```python
from build123d import *

# Parameters (mm, degrees)
BOSS_EXTRUDE1_DEPTH   = 27.432
BOSS_EXTRUDE2_DEPTH   = 5.08
SKETCH4_R             = 1.524
CUT_EXTRUDE1_DEPTH    = 2.286
SKETCH4_4_R           = 1.524
CUT_EXTRUDE2_DEPTH    = 63.630575033
BOSS_EXTRUDE3_DEPTH   = 3.81
FILLET1_R             = 2.54
CHAMFER3_SIZE         = 1.27
CHAMFER4_SIZE         = 0.254
SKETCH8_W             = 101.6
SKETCH8_H             = 44.45
CUT_EXTRUDE3_DEPTH    = 5.08
CHAMFER5_SIZE         = 1.27
BOSS_EXTRUDE4_DEPTH   = 6.096
FILLET2_R             = 1.27
CUT_EXTRUDE4_DEPTH    = 15.24
MIRROR3_COPY_1_DEPTH  = 15.24
CHAMFER7_SIZE         = 0.381
SKETCH19_W            = 135.869666512
SKETCH19_H            = 67.345799606
CUT_EXTRUDE9_DEPTH    = 31.242
BOSS_EXTRUDE6_DEPTH   = 20.32
SKETCH21_W            = 80.01
SKETCH21_H            = 52.07
BOSS_EXTRUDE7_DEPTH   = 3.81
FILLET3_R             = 2.54
CHAMFER8_SIZE         = 1.27
BOSS_EXTRUDE8_DEPTH   = 10.16
BOSS_EXTRUDE10_DEPTH  = 5.08
MIRROR13_COPY_1_DEPTH = 10.16
MIRROR13_COPY_2_DEPTH = 5.08
SKETCH27_W            = 107.092264377
SKETCH27_H            = 185.22400122
CUT_EXTRUDE11_DEPTH   = 177.054251014
SKETCH28_W            = 133.557103753
SKETCH28_H            = 91.2241148
CUT_EXTRUDE12_DEPTH   = 45.72


with BuildPart() as part:
    # Sketch1 → Boss-Extrude1 (new body)
    with BuildSketch(Plane(origin=(10.858740921, 0, 0), x_dir=(1, 0, 0), z_dir=(0, 0, 1))):
        Polygon((-52.705, 25.4), (-52.705, 21.59), (48.895, 21.59), (48.895, -22.86), (-52.705, -22.86), (-52.705, -25.4), (52.705, -25.4), (52.705, 25.4), align=None)
    extrude(amount=BOSS_EXTRUDE1_DEPTH)

    # Sketch1<3> → Boss-Extrude2 (add)
    with BuildSketch(Plane(origin=(10.858740921, 0, 0), x_dir=(1, 0, 0), z_dir=(0, 0, 1))):
        Polygon((48.895, 21.59), (-52.705, 21.59), (-52.705, 13.97), (-6.985, 13.97), (-6.985, -6.35), (-52.705, -6.35), (-52.705, -22.86), (48.895, -22.86), align=None)
    extrude(amount=BOSS_EXTRUDE2_DEPTH)

    # Sketch4 → Cut-Extrude1 (cut)
    # profile 1 of 4: a face of its own
    with BuildSketch(Plane(origin=(10.858740921, 0, 5.08), x_dir=(1, 0, 0), z_dir=(0, 0, 1))):
        Polygon((-44.785877438, 21.59), (-47.924122562, 21.59), (-49.493245123, 18.8722), (-47.924122562, 16.1544), (-44.785877438, 16.1544), (-43.216754877, 18.8722), align=None)
        with Locations((-46.355, 18.8722)):
            Circle(SKETCH4_R, mode=Mode.SUBTRACT)
    # profile 2 of 4: a face of its own
    with BuildSketch(Plane(origin=(10.858740921, 0, 5.08), x_dir=(1, 0, 0), z_dir=(0, 0, 1))):
        Polygon((21.126640721, 16.1544), (17.988395597, 16.1544), (16.419273036, 18.8722), (17.988395597, 21.59), (21.126640721, 21.59), (22.695763282, 18.8722), align=None)
        with Locations((19.557518159, 18.8722)):
            Circle(SKETCH4_R, mode=Mode.SUBTRACT)
    # profile 3 of 4: a face of its own
    with BuildSketch(Plane(origin=(10.858740921, 0, 5.08), x_dir=(1, 0, 0), z_dir=(0, 0, 1))):
        Polygon((22.695763282, -18.8722), (21.126640721, -16.1544), (17.988395597, -16.1544), (16.419273036, -18.8722), (17.988395597, -21.59), (21.126640721, -21.59), align=None)
        with Locations((19.557518159, -18.8722)):
            Circle(SKETCH4_R, mode=Mode.SUBTRACT)
    # profile 4 of 4: a face of its own
    with BuildSketch(Plane(origin=(10.858740921, 0, 5.08), x_dir=(1, 0, 0), z_dir=(0, 0, 1))):
        Polygon((-49.493245123, -18.8722), (-47.924122562, -16.1544), (-44.785877438, -16.1544), (-43.216754877, -18.8722), (-44.785877438, -21.59), (-47.924122562, -21.59), align=None)
        with Locations((-46.355, -18.8722)):
            Circle(SKETCH4_R, mode=Mode.SUBTRACT)
    extrude(amount=-CUT_EXTRUDE1_DEPTH, mode=Mode.SUBTRACT)

    # Sketch4<4> → Cut-Extrude2 (cut, through all)
    with BuildSketch(Plane(origin=(10.858740921, 0, 5.08), x_dir=(1, 0, 0), z_dir=(0, 0, 1))):
        with Locations((-46.355, 18.8722)):
            Circle(SKETCH4_4_R)
        with Locations((19.557518159, 18.8722)):
            Circle(SKETCH4_4_R)
        with Locations((-46.355, -18.8722)):
            Circle(SKETCH4_4_R)
        with Locations((19.557518159, -18.8722)):
            Circle(SKETCH4_4_R)
    extrude(amount=-CUT_EXTRUDE2_DEPTH, mode=Mode.SUBTRACT)

    # Sketch7 → Boss-Extrude3 (add)
    with BuildSketch(Plane(origin=(10.858740921, 0, 27.432), x_dir=(1, 0, 0), z_dir=(0, 0, 1))):
        Polygon((-52.705, 25.4), (52.705, 25.4), (52.705, -25.4), (-52.705, -25.4), (-52.705, -6.35), (-46.355, -6.35), (-46.355, 6.35), (-52.705, 6.35), align=None)
    extrude(amount=BOSS_EXTRUDE3_DEPTH)

    # Fillet1
    fillet1_edges = [part.edges().sort_by_distance(p)[0] for p in [
        (63.563740921, 25.4, 15.621),
        (63.563740921, -25.4, 15.621),
        (10.858740921, -25.4, 31.242),
        (63.563740921, 0, 31.242),
        (10.858740921, 25.4, 31.242),
    ]]
    fillet(fillet1_edges, radius=FILLET1_R)

    # Chamfer3
    chamfer3_edges = [part.edges().sort_by_distance(p)[0] for p in [
        (-41.846259079, 13.97, 27.432),
        (-41.846259079, 6.35, 29.337),
        (-41.846259079, 21.59, 16.256),
        (-41.846259079, -14.605, 27.432),
        (-41.846259079, -6.35, 29.337),
        (-38.671259079, 6.35, 31.242),
        (-35.496259079, 0, 31.242),
        (-38.671259079, -6.35, 31.242),
        (-41.846259079, -22.86, 16.256),
    ]]
    chamfer(chamfer3_edges, length=CHAMFER3_SIZE)

    # Chamfer4
    chamfer4_edges = [part.edges().sort_by_distance(p)[0] for p in [
        (28.892259079, 18.8722, 0),
        (-37.020259079, -18.8722, 0),
        (28.892259079, -18.8722, 0),
        (-37.020259079, 18.8722, 0),
    ]]
    chamfer(chamfer4_edges, length=CHAMFER4_SIZE)

    # Sketch8 → Cut-Extrude3 (cut)
    with BuildSketch(Plane(origin=(10.858740921, 0, 5.08), x_dir=(1, 0, 0), z_dir=(0, 0, 1))):
        with Locations((-1.905, -0.635)):
            Rectangle(SKETCH8_W, SKETCH8_H)
    extrude(amount=-CUT_EXTRUDE3_DEPTH, mode=Mode.SUBTRACT)

    # Chamfer5
    chamfer5_edges = [part.edges().sort_by_distance(p)[0] for p in [
        (-41.846259079, -22.86, 2.54),
        (-41.846259079, 21.59, 2.54),
    ]]
    chamfer(chamfer5_edges, length=CHAMFER5_SIZE)

    # Sketch9 → Boss-Extrude4 (add)
    with BuildSketch(Plane(origin=(10.858740921, 0, 0), x_dir=(-1, 0, 0), z_dir=(0, 0, -1))):
        Polygon((-90.741259079, 28.1), (-80.741259079, 38.1), (102.458740921, 38.1), (112.458740921, 28.1), (112.458740921, -28.1), (102.458740921, -38.1), (-80.741259079, -38.1), (-90.741259079, -28.1), align=None)
    extrude(amount=BOSS_EXTRUDE4_DEPTH)

    # Fillet2
    fillet2_edges = [part.edges().sort_by_distance(p)[0] for p in [
        (9.588740921, -25.4, 0),
        (63.563740921, 0, 0),
        (9.588740921, 25.4, 0),
        (62.819792145, 24.656051224, 0),
        (62.819792145, -24.656051224, 0),
    ]]
    fillet(fillet2_edges, radius=FILLET2_R)

    # Sketch13 → Cut-Extrude4 (cut)
    with BuildSketch(Plane(origin=(-64.85, 64.85, 0), x_dir=(0, 0, 1), z_dir=(-0.7071067811865477, 0.7071067811865474, 0))):
        Polygon((-6.096, -44.901280605), (-6.096, -42.070807846), (0, -38.551280605), (0, -51.251280605), (-6.096, -47.731753364), align=None)
    cut_extrude4 = extrude(amount=-CUT_EXTRUDE4_DEPTH, mode=Mode.SUBTRACT)

    # Mirror2: Cut-Extrude4 across plane
    add(cut_extrude4.mirror(Plane.ZX), mode=Mode.SUBTRACT)

    # Mirror3: Cut-Extrude4 across plane
    add(cut_extrude4.mirror(Plane(origin=(0, 0, 0), x_dir=(0, 0, 1), z_dir=(1, 0, 0))), mode=Mode.SUBTRACT)

    # Mirror3 copy 1 sketch → Mirror3 copy 1 (cut)
    with BuildSketch(Plane(origin=(64.85, -64.85, 0), x_dir=(0, 0, 1), z_dir=(0.7071067811865477, -0.7071067811865474, 0))):
        Polygon((-6.096, -44.901280605), (-6.096, -42.070807846), (0, -38.551280605), (0, -51.251280605), (-6.096, -47.731753364), align=None)
    extrude(amount=-MIRROR3_COPY_1_DEPTH, mode=Mode.SUBTRACT)

    # Chamfer7
    chamfer7_edges = [part.edges().sort_by_distance(p)[0] for p in [
        (-99.845787271, 29.854212729, -3.048),
        (-93.354212729, 36.345787271, -3.048),
        (-99.845787271, -29.854212729, -3.048),
        (-93.354212729, -36.345787271, -3.048),
        (99.845787271, 29.854212729, -3.048),
        (93.354212729, 36.345787271, -3.048),
        (99.845787271, -29.854212729, -3.048),
        (93.354212729, -36.345787271, -3.048),
    ]]
    chamfer(chamfer7_edges, length=CHAMFER7_SIZE)

    # Sketch19 → Cut-Extrude9 (cut)
    with BuildSketch(Plane.XY.offset(31.242)):
        Rectangle(SKETCH19_W, SKETCH19_H)
    extrude(amount=-CUT_EXTRUDE9_DEPTH, mode=Mode.SUBTRACT)

    # Sketch20 → Boss-Extrude6 (add)
    with BuildSketch(Plane.XY):
        Polygon((65.405, 22.86), (65.405, -21.59), (-10.795, -21.59), (-10.795, -25.4), (69.215, -25.4), (69.215, 26.67), (-10.795, 26.67), (-10.795, 22.86), align=None)
    extrude(amount=BOSS_EXTRUDE6_DEPTH)

    # Sketch21 → Boss-Extrude7 (add)
    with BuildSketch(Plane.XY.offset(20.32)):
        with Locations((29.21, 0.635)):
            Rectangle(SKETCH21_W, SKETCH21_H)
    extrude(amount=BOSS_EXTRUDE7_DEPTH)

    # Fillet3
    fillet3_edges = [part.edges().sort_by_distance(p)[0] for p in [
        (29.21, -25.4, 0),
        (69.215, 0.635, 0),
        (69.215, -25.4, 12.065),
        (29.21, 26.67, 0),
        (69.215, 26.67, 12.065),
        (29.21, -25.4, 24.13),
        (69.215, 0.635, 24.13),
        (29.21, 26.67, 24.13),
    ]]
    fillet(fillet3_edges, radius=FILLET3_R)

    # Chamfer8
    chamfer8_edges = [part.edges().sort_by_distance(p)[0] for p in [
        (-10.795, 22.86, 10.16),
        (-10.795, -21.59, 10.16),
        (-10.795, 0.635, 20.32),
    ]]
    chamfer(chamfer8_edges, length=CHAMFER8_SIZE)

    # Sketch24 → Boss-Extrude8 (add)
    with BuildSketch(Plane.XY):
        Polygon((-90.762833521, 19.180603012), (-101.6, 8.343436534), (-101.6, 28.1), (-100.641115254, 29.058884746), align=None)
        Polygon((-92.558884746, 37.141115254), (-91.6, 38.1), (-71.843436534, 38.1), (-82.680603012, 27.262833521), align=None)
    boss_extrude8 = extrude(amount=BOSS_EXTRUDE8_DEPTH)

    # Sketch26 → Boss-Extrude10 (add)
    with BuildSketch(Plane.XY.offset(10.16)):
        Polygon((-101.6, 8.343436534), (-71.843436534, 38.1), (-91.6, 38.1), (-101.6, 28.1), align=None)
    boss_extrude10 = extrude(amount=BOSS_EXTRUDE10_DEPTH)

    # Mirror12: Boss-Extrude8, Boss-Extrude10 across plane
    add(boss_extrude8.mirror(Plane.ZX))
    add(boss_extrude10.mirror(Plane.ZX))

    # Mirror13: Boss-Extrude8, Boss-Extrude10 across plane
    add(boss_extrude8.mirror(Plane(origin=(0, 0, 0), x_dir=(0, 0, 1), z_dir=(1, 0, 0))))
    add(boss_extrude10.mirror(Plane(origin=(0, 0, 0), x_dir=(0, 0, 1), z_dir=(1, 0, 0))))

    # Mirror13 copy 1 sketch → Mirror13 copy 1 (add)
    with BuildSketch(Plane(origin=(0, 0, 0), x_dir=(-1, 0, 0), z_dir=(0, 0, 1))):
        Polygon((-90.762833521, 19.180603012), (-101.6, 8.343436534), (-101.6, 28.1), (-100.641115254, 29.058884746), align=None)
        Polygon((-92.558884746, 37.141115254), (-91.6, 38.1), (-71.843436534, 38.1), (-82.680603012, 27.262833521), align=None)
    extrude(amount=MIRROR13_COPY_1_DEPTH)

    # Mirror13 copy 2 sketch → Mirror13 copy 2 (add)
    with BuildSketch(Plane(origin=(0, 0, 10.16), x_dir=(-1, 0, 0), z_dir=(0, 0, 1))):
        Polygon((-101.6, 8.343436534), (-71.843436534, 38.1), (-91.6, 38.1), (-101.6, 28.1), align=None)
    extrude(amount=MIRROR13_COPY_2_DEPTH)

    # Sketch27 → Cut-Extrude11 (cut, through all)
    with BuildSketch(Plane.ZY.offset(68.58)):
        with Locations((3.455221188, 0)):
            Rectangle(SKETCH27_W, SKETCH27_H)
    extrude(amount=-CUT_EXTRUDE11_DEPTH, mode=Mode.SUBTRACT)

    # Sketch28 → Cut-Extrude12 (cut)
    with BuildSketch(Plane.XZ.offset(38.1)):
        with Locations((-79.914224937, 5.971845756)):
            Rectangle(SKETCH28_W, SKETCH28_H)
    extrude(amount=-CUT_EXTRUDE12_DEPTH, mode=Mode.SUBTRACT)


solid = part.part
```
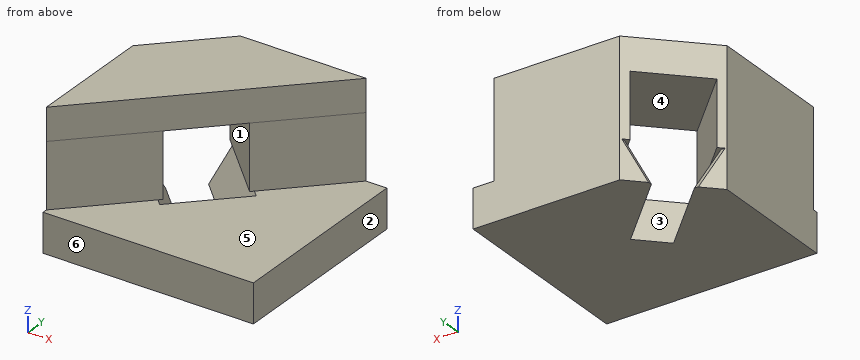
Work out the finished part from the listing and answer in its coordinate system (mm). Face numbers are marked on the shaded views. A direction names the side the tool comes from. Give positions to 0.01 mm unless a question says otherwise; leave off trailing zeros. Order: outer loops, then holes, each group sorted by start corner. A loop starts at its lowest first (then second) coordinate and runs counter-clockwise, first axis right, second up. Notation, with made-up numbers: M -18.75,24 L 30.25,24 A10 ccw 30.25,40 Z; hole C 37.25,28.5 d7. An arc over 180 degrees is marked long. Return JSON: item names as keys, results as strings.
1) A tool of negligible diameter and unlimited length cuts with its end or side. For the marked faces 1, 2 and 3, from which of +Z, -Z, +X, -X, +Y, -Y can it reach the whole face along a straight path? Write none if from no direction.
Resolved:
{"face 1": "none", "face 2": "+Z, -Z, +X, +Y, -Y", "face 3": "+Z"}
2) For a pull along Y with two mould halves and no side action, classify the marked faces 4, 5 and 6 as +Y half, -Y half, draft (parallel to the pull), parting line (faces both ways), or undercut.
Resolved:
{"face 4": "undercut", "face 5": "draft", "face 6": "-Y half"}
3) Each of these flat-tipped pins is pushed along its axis until it touches: pin 1 (2 mm diameter, centred on y = 19, z = 12.5, fed in from +X); pin 2 (12 mm diameter, centred on x = -87.5, z = 10, fed in from -Y); pin 3 (3 mm diameter, centred on y = 12.5, z = 11.5, fed in from +X). Where does it stop, or does it pass through?
Resolved:
{"pin 1": "x = -89.94", "pin 2": "y = 16.44", "pin 3": "x = -95.94"}
4) Section C-C, the plane y = 21 is taken. Write down the section's boundary in (x, z), plus the area to 3 significant figures.
Resolved:
{"outline": "M -101.6,-6.1 L -88.5,-6.1 L -93.48,0 L -92.58,0 L -92.58,10.16 L -88.94,10.16 L -88.94,15.24 L -101.6,15.24 Z; M -87.15,-6.1 L -68.58,-6.1 L -68.58,0 L -87.15,0 Z", "area": "334 mm^2"}
5) Section D-D, the plane x = -78 is taken. Write down the section's boundary in (y, z).
Resolved:
{"outline": "M 7.62,-6.1 L 38.1,-6.1 L 38.1,15.24 L 31.94,15.24 L 31.94,0 L 7.62,0 Z"}
6) Section B-B, the plane x = -88.5 is taken. Write down the section's boundary in (y, z).
Resolved:
{"outline": "M 7.62,-6.1 L 21,-6.1 L 19.65,-4.44 L 19.65,0 L 7.62,0 Z; M 21.44,10.16 L 33.08,10.16 L 33.08,0 L 33.98,0 L 29,-6.1 L 38.1,-6.1 L 38.1,15.24 L 21.44,15.24 Z"}
7) Section A-A, the plane z = 1 is taken. Write down the section's boundary in (x, y).
Resolved:
{"outline": "M -101.6,8.34 L -90.76,19.18 L -100.64,29.06 L -101.6,28.1 Z; M -92.56,37.14 L -82.68,27.26 L -71.84,38.1 L -91.6,38.1 Z"}
8) Straight lines are drawn through the part: line 1 along Z through (x, y) = (-95, 11); line 2 along Z through (x, y) = (-90.5, 30.5); line 3 along Z through (x, y) = (-95, 27). For each, find the intervals that lie inside material, in ascending order. Write a range as [from, to].
Resolved:
{"line 1": "[-6.1, 0]", "line 2": "[10.16, 15.24]", "line 3": "[-6.1, -5.49], [10.16, 15.24]"}
